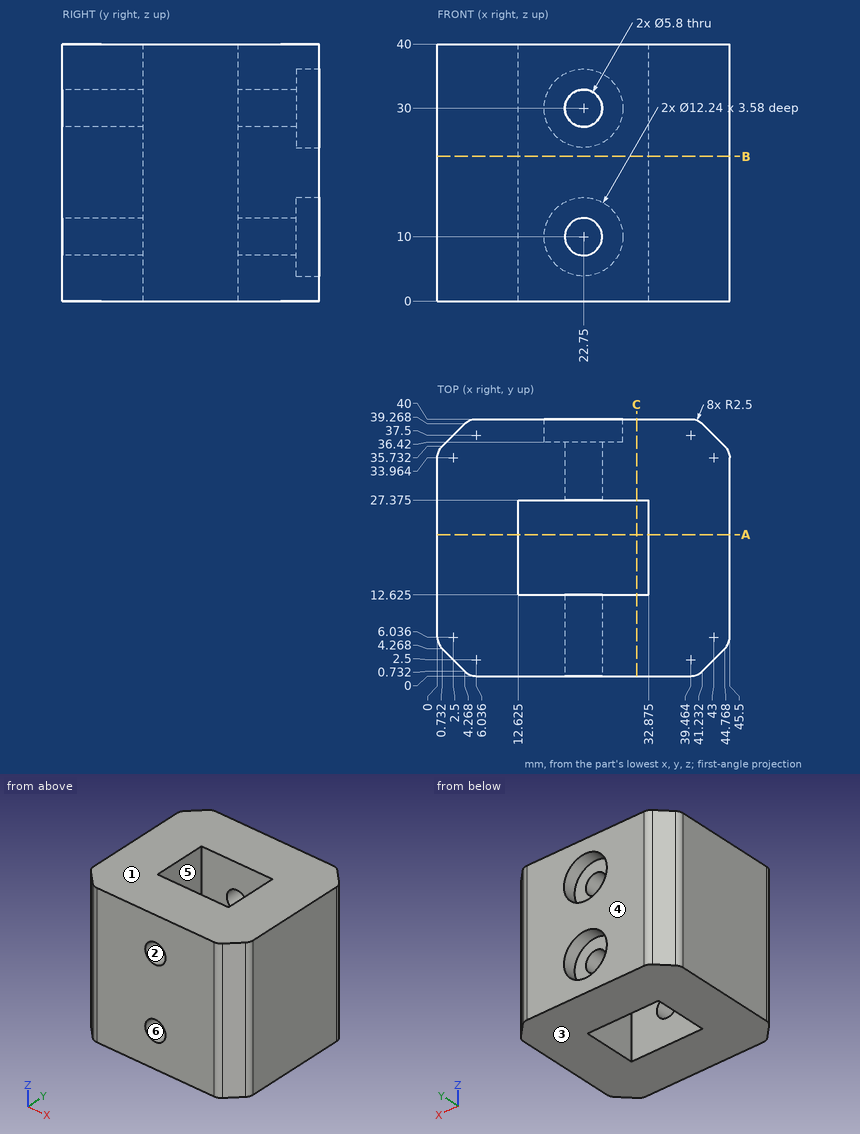
For this review, use the dimensioned drawing (mm, ordinates from the lowest corner) and the shaded views. A direction names the side the tool comes from. Give positions to 0.01 mm unless a question says otherwise; leave off trailing zeros. Order: outer loops, then holes, each group sorted by start corner. A loop starts at its lowest first (then second) coordinate and runs counter-clockwise, first axis right, second up. Notation, with made-up numbers: (4, -24) - (56, -24) arc R24 cw to (56, 15) - close; hole circle Ø2 at (-27.5, 18.25). An arc over 180 degrees is marked (long way). Use a Markdown table: item, result. Add a question column.
(1) Mouldability with a two-part tool opening along Z and no side actions: class the marked faces 1, 2, 3 and 4 as +Z half, -Z half, draft (parallel to the pull), parting line (faces both ways), or undercut.
(2) Add section A-A on y = 22. Give the boundary of the cut face in (x, z) (1 decimal), then the cut area to 3 significant figures.
(3) Add section B-B on z = 22.5. Give the boundary of the cut face in (x, y) (1 decimal), then the cut area to 3 significant figures.
(4) Wall thickness on probe 1 along Z at (x, y) = (22.75, 34.25); probe 2 along Y at (x, z) = (26.5, 37) (1 decimal); probe 3 along X at (y, z) = (31.25, 10): over which ranges is each line inside the solid? List them lowest first. Write a range as [from, to].
(5) Add section C-C on x = 31. Give the boundary of the cut face in (y, z) (1 decimal).
(6) Clearance check with a flat-ended pin moving along its axis: P1, Ø6, axis at x = 20.5, z = 30, coming from the +Y side. State where the tip first meets the part, or that it passes through.
(7) Machinability: for the marked faces 5 and 6, which of the approach directions +Z, -Z, +X, -X, +Y, -Y give a long, thin tool a straight path to every point of the face, cutting with its end or side? Answer none if there is none.
Report:
| question | item | result |
|---|---|---|
| 1 | face 1 | +Z half |
| 1 | face 2 | undercut |
| 1 | face 3 | -Z half |
| 1 | face 4 | draft |
| 2 | outline | (0, 0) - (12.6, 0) - (12.6, 40) - (0, 40) - close; (32.9, 0) - (45.5, 0) - (45.5, 40) - (32.9, 40) - close |
| 2 | area | 1,010 mm² |
| 3 | outline | (0, 6) arc R2.5 ccw to (0.7, 4.3) - (4.3, 0.7) arc R2.5 ccw to (6, 0) - (39.5, 0) arc R2.5 ccw to (41.2, 0.7) - (44.8, 4.3) arc R2.5 ccw to (45.5, 6) - (45.5, 34) arc R2.5 ccw to (44.8, 35.7) - (41.2, 39.3) arc R2.5 ccw to (39.5, 40) - (6, 40) arc R2.5 ccw to (4.3, 39.3) - (0.7, 35.7) arc R2.5 ccw to (0, 34) - close; hole (12.6, 12.6) - (32.9, 12.6) - (32.9, 27.4) - (12.6, 27.4) - close |
| 3 | area | 1,470 mm² |
| 4 | probe 1 | z = [0, 7.1], [12.9, 27.1], [32.9, 40] |
| 4 | probe 2 | y = [0, 12.6], [27.4, 40] |
| 4 | probe 3 | x = [0, 19.85], [25.65, 45.5] |
| 5 | outline | (0, 0) - (12.6, 0) - (12.6, 40) - (0, 40) - close; (27.4, 0) - (40, 0) - (40, 40) - (27.4, 40) - close |
| 6 | P1 | stops at y = 36.42 |
| 7 | face 5 | +Z, -Z |
| 7 | face 6 | +Y, -Y |
